Verification items for the finished model (mm, model axes). A direction names the side the tool comes from. Coordinates: 2 decimals unless noted, no trailing zeros. Write each loop counter-clockwise with the first axis right and the second up, starting at its lowest first coordinate (ties: lowest second). Pieces come first, ordered by that corner, then holes. Notation, with made-up numbers: (73, 77.25) -> (99, 77.25) arc R19 cw to (99, 86.25) -> close; hole circle Ø9 at (1, -34). An arc over 180 degrees is marked (long way). Answer in a Markdown table with one row per item.
```python
from build123d import *

# Parameters (mm, degrees)
BOSS_EXTRUDE1_DEPTH = 100
SKETCH2_R           = 52.5
BOSS_EXTRUDE2_DEPTH = 400
BOSS_EXTRUDE3_START = -400
BOSS_EXTRUDE3_DEPTH = 400
SKETCH4_W           = 56.007810594
SKETCH4_H           = 50
BOSS_EXTRUDE4_DEPTH = 1050


with BuildPart() as part:
    # Sketch1 → Boss-Extrude1 (new body)
    with BuildSketch(Plane.XY):
        Polygon((-1000, 200), (-900, 200), (-900, -200), (-1000, -200), (-1000, -250), (1000, -250), (1000, -200), (900, -200), (900, 200), (1000, 200), (1000, 250), (-1000, 250), align=None)
    extrude(amount=BOSS_EXTRUDE1_DEPTH)

    # Sketch2 → Boss-Extrude2 (add)
    with BuildSketch(Plane.XZ.offset(-200)):
        with Locations(Location((960, 50, 0), (0, 0, 107.752790162))):
            Circle(SKETCH2_R)
    boss_extrude2 = extrude(amount=BOSS_EXTRUDE2_DEPTH)

    # Mirror1: Boss-Extrude2 across plane
    add(boss_extrude2.mirror(Plane(origin=(0, 0, 0), x_dir=(0, 0, 1), z_dir=(1, 0, 0))))

    # Sketch3 → Boss-Extrude3 (add)
    with BuildSketch(Plane.XZ.offset(200).offset(BOSS_EXTRUDE3_START)):
        with BuildLine():
            Line((959.98965758, -4.499999019), (-1002.277476215, 15.607195449))
            ThreePointArc((-1002.277476215, 15.607195449), (-1009.217160869, 73.407714027), (-960, 104.5))
            Line((-960, 104.5), (960, 104.5))
            ThreePointArc((960, 104.5), (1014.499999755, 49.99482879), (959.98965758, -4.499999019))
        make_face()
        with BuildLine():
            Line((-960, 102.5), (960, 102.5))
            ThreePointArc((960, 102.5), (1012.5, 50), (960, -2.5))
            Line((960, -2.5), (-1001.307615203, 17.597362357))
            ThreePointArc((-1001.307615203, 17.597362357), (-1007.209048265, 72.96858206), (-960, 102.5))
        make_face(mode=Mode.SUBTRACT)
    extrude(amount=BOSS_EXTRUDE3_DEPTH)

    # Sketch4 → Boss-Extrude4 (add)
    with BuildSketch(Plane(origin=(0, 0, 0), x_dir=(-1, 0, 0), z_dir=(0, 0, -1))):
        with Locations((-971.996094703, 225)):
            Rectangle(SKETCH4_W, SKETCH4_H)
        with Locations((971.996094703, 225)):
            Rectangle(SKETCH4_W, SKETCH4_H)
        with Locations((971.996094703, -225)):
            Rectangle(SKETCH4_W, SKETCH4_H)
        with Locations((-971.996094703, -225)):
            Rectangle(SKETCH4_W, SKETCH4_H)
    extrude(amount=BOSS_EXTRUDE4_DEPTH)


solid = part.part
```
1. Section check A-A, the plane x = 477.5. Record the boundary of the cut face in (y, z), plus the area to 3 significant figures.
Geometry says:
| item | result |
|---|---|
| outline | (-250, 0) -> (250, 0) -> (250, 100) -> (-250, 100) -> close; (-200, 102.5) -> (200, 102.5) -> (200, 104.5) -> (-200, 104.5) -> close |
| area | 50,800 mm^2 |
2. Tool access check on faces 1 (the flat face through (79, 250, 39)), 2 (the flat face through (-900, 3, 58)), 3 (the flat face through (-943.992, 225, -518)). Record the directions out of +Z, -Z, +X, -X, +Y, -Y that give a thin tool (end or side, any length) a straight path to the whole face; none if there is none.
Geometry says:
| item | result |
|---|---|
| face 1 | +Z, -Z, +X, -X, +Y |
| face 2 | none |
| face 3 | -Z, +Y, -Y |
3. Depth check by flat-ended pin: P1, Ø4.5, axis at y = -67, z = 8, coming from the -X side; P2, Ø4, axis at x = -688, y = -25.5, coming from the -Z side; P3, Ø15, axis at y = -216, z = -342.5, coming from the -X side. Enter the tip coordinate at first touch or a pass-through.
Geometry says:
| item | result |
|---|---|
| P1 | x = -994.3 |
| P2 | z = 0 |
| P3 | x = -1000 |
4. Thickness scan on line 1 (X direction, y = 224.5, z = -385.5); line 2 (Z direction, x = 203, y = -17); line 3 (X direction, y = 94.5, z = 58). Record the ranges inside material, lowest first. Write a range as from..to.
Geometry says:
| item | result |
|---|---|
| line 1 | -1000..-943.99, 943.99..1000 |
| line 2 | 0..100, 102.5..104.5 |
| line 3 | -1013.91..-908.11, -900..900, 908.11..1013.91 |
5. Section check C-C, the plane z = -736. Record the boundary of the cut face in (x, y), plus the area to 3 significant figures.
Geometry says:
| item | result |
|---|---|
| outline | (-1000, -250) -> (-943.99, -250) -> (-943.99, -200) -> (-1000, -200) -> close; (-1000, 200) -> (-943.99, 200) -> (-943.99, 250) -> (-1000, 250) -> close; (943.99, -250) -> (1000, -250) -> (1000, -200) -> (943.99, -200) -> close; (943.99, 200) -> (1000, 200) -> (1000, 250) -> (943.99, 250) -> close |
| area | 11,200 mm^2 |
6. Mould release check, pull along Z, two halves, no side actions. Record for faces 4 (the flat face through (-13, 3, 102.5)), 5 (the flat face through (1000, 225, -467)), 6 (the cylindrical face through (-1009.58, 2.8, 72.63)): released by +Z, released by -Z, zero draft, split by the parting line, or undercut.
Geometry says:
| item | result |
|---|---|
| face 4 | undercut |
| face 5 | zero draft |
| face 6 | split by the parting line |
7. Section check B-B, the plane y = 8.5. Record the boundary of the cut face in (x, z), plus the area to 3 significant figures.
Geometry says:
| item | result |
|---|---|
| outline | (-1002.28, 15.61) -> (-999.64, 15.58) arc R52.5 ccw to (-921.07, 14.78) -> (-900, 14.56) -> (-900, 0) -> (520.83, 0) -> (959.99, -4.5) arc R54.5 ccw to (960, 104.5) -> (-960, 104.5) arc R54.5 ccw to start; hole (-960, 102.5) arc R52.5 cw to (-919.37, 16.76) -> (-900, 16.56) -> (-900, 100) -> (900, 100) -> (900, 0) -> (716.02, 0) -> (958.92, -2.49) arc R52.5 cw to (960, 102.5) -> close |
| area | 202,000 mm^2 |
